For this review, take the finished solid that the model builds, in its own axes (mm). Face numbers are marked on the shaded views. Give positions to 0.01 mm unless a question says otherwise; leave off trailing zeros. Order: outer loops, then holes, each group sorted by start corner. A loop starts at its lowest first (then second) coordinate and runs counter-clockwise, first axis right, second up. Notation, with made-up numbers: M -34.5,21 L 15.5,21 A30 ccw 15.5,60 Z; hole C -4.75,11 d5. An arc over 180 degrees is marked long. Use CSV: the item, a comma, the result in double quotes. Start each with the question number.
(1) Clearance check with flat-ended pins moving along their axes: P1, Ø1.6, axis at x = -85.5, z = 3, coming from the -Y side; P2, Ø2.5, axis at x = 146, z = 2.5, coming from the +Y side; P3, Ø6, axis at x = 94, y = 28.5, coming from the -Z side; P4, Ø1.8, axis at x = -133.5, z = 1.5, coming from the +Y side. State where each tip first meets the part, or that it passes through.
(2) Wall thickness on L1, parallel to X at y = 31.5, z = 1.3; L2, parallel to X at y = 53, z = 4.7; L3, parallel to X at y = 70, z = 1.5: over which ranges is each line inside the solid? List them lowest first. Write a range as from..to.
(3) Consider section C-C (z = 3.8). Give the number of separate pieces and of enclosed holes in the cut face, and give its area (3 significant figures).
(4) Draft analysis for pull direction Z (two halves, no side actions). For the marked faces 1 and 2, state which applies: pulls with the +Z half, pulls with the -Z half, needs draft (parallel to the pull), parting line crosses it, or undercut.
(5) Consider section A-A (y = 11.5). Write out the cut boundary in (x, z), and give its area (3 significant figures).
(6) Consider section B-B (x = -23). Write out the cut boundary in (y, z), and give its area (3 significant figures).
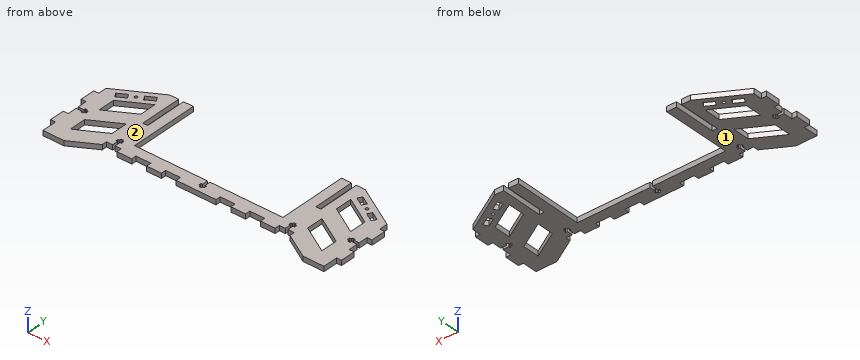
```python
from build123d import *

# Parameters (mm, degrees)
ESTRUSIONE_ESTRUSIONE1_DEPTH = 5
SCHIZZO2_R                   = 1.5
TAGLIO_ESTRUSIONE2_DEPTH     = 6
SCHIZZO5_W                   = 15
SCHIZZO5_H                   = 5
SCHIZZO5_W_2                 = 5
SCHIZZO5_H_2                 = 42.5
SCHIZZO5_W_3                 = 150.358983848
SCHIZZO5_H_3                 = 70
TAGLIO_ESTRUSIONE3_DEPTH     = 6
TAGLIO_ESTRUSIONE4_DEPTH     = 6
SCHIZZO7_R                   = 0.25
TAGLIO_ESTRUSIONE5_DEPTH     = 10


with BuildPart() as part:
    # Schizzo1 → Estrusione-Estrusione1 (new body)
    with BuildSketch(Plane.XY):
        Polygon((-142.5, 75), (-142.5, 66.339745962), (-147.5, 66.339745962), (-147.5, 51.339745962), (-142.5, 51.339745962), (-142.5, 30), (-147.5, 30), (-147.5, 15), (-142.5, 15), (-142.5, 0), (142.5, 0), (142.5, 15), (147.5, 15), (147.5, 30), (142.5, 30), (142.5, 51.339745962), (147.5, 51.339745962), (147.5, 66.339745962), (142.5, 66.339745962), (142.5, 75), (99.198729811, 100), (-99.198729811, 100), align=None)
    extrude(amount=ESTRUSIONE_ESTRUSIONE1_DEPTH)

    # Schizzo2 → Taglio-Estrusione2 (cut, through all)
    with BuildSketch(Plane.XY):
        with Locations((-117.099364905, 81.004809472)):
            Circle(SCHIZZO2_R)
        with Locations((117.099364905, 81.004809472)):
            Circle(SCHIZZO2_R)
        Polygon((-99.198729811, 82.679491924), (-127.5, 66.339745962), (-127.5, 49.330127019), (-99.198729811, 65.669872981), align=None)
        Polygon((99.198729811, 31.339745962), (99.198729811, 48.349364905), (127.5, 32.009618943), (127.5, 15), align=None)
        Polygon((-95.179491924, 15), (-121.160254038, 0), (121.160254038, 0), (95.179491924, 15), align=None)
        Polygon((-99.198729811, 31.339745962), (-127.5, 15), (-127.5, 32.009618943), (-99.198729811, 48.349364905), align=None)
        Polygon((99.198729811, 65.669872981), (99.198729811, 82.679491924), (127.5, 66.339745962), (127.5, 49.330127019), align=None)
        Polygon((-132.5, 75), (-123.839745962, 80), (-121.339745962, 75.669872981), (-130, 70.669872981), align=None)
        Polygon((-104.198729811, 91.339745962), (-101.698729811, 87.009618943), (-110.358983849, 82.009618943), (-112.858983849, 86.339745962), align=None)
        Polygon((132.5, 75), (130, 70.669872981), (121.339745962, 75.669872981), (123.839745962, 80), align=None)
        Polygon((104.198729811, 91.339745962), (112.858983849, 86.339745962), (110.358983849, 82.009618943), (101.698729811, 87.009618943), align=None)
    extrude(amount=TAGLIO_ESTRUSIONE2_DEPTH, mode=Mode.SUBTRACT)

    # Schizzo5 → Taglio-Estrusione3 (cut, through all)
    with BuildSketch(Plane.XY):
        with Locations((-87.679491924, 17.5)):
            Rectangle(SCHIZZO5_W, SCHIZZO5_H)
        with Locations((-57.679491924, 17.5)):
            Rectangle(SCHIZZO5_W, SCHIZZO5_H)
        with Locations((-27.679491924, 17.5)):
            Rectangle(SCHIZZO5_W, SCHIZZO5_H)
        with Locations((27.679491924, 17.5)):
            Rectangle(SCHIZZO5_W, SCHIZZO5_H)
        with Locations((57.679491924, 17.5)):
            Rectangle(SCHIZZO5_W, SCHIZZO5_H)
        with Locations((87.679491924, 17.5)):
            Rectangle(SCHIZZO5_W, SCHIZZO5_H)
        with Locations((87.679491924, 78.75)):
            Rectangle(SCHIZZO5_W_2, SCHIZZO5_H_2)
        with Locations((-87.679491924, 78.75)):
            Rectangle(SCHIZZO5_W_2, SCHIZZO5_H_2)
        with Locations((0, 65)):
            Rectangle(SCHIZZO5_W_3, SCHIZZO5_H_3)
    extrude(amount=TAGLIO_ESTRUSIONE3_DEPTH, mode=Mode.SUBTRACT)

    # Schizzo6 → Taglio-Estrusione4 (cut, through all)
    with BuildSketch(Plane.XY):
        Polygon((-142.5, 41.919872981), (-136.5, 41.919872981), (-136.5, 43.419872981), (-134.1, 43.419872981), (-134.1, 41.919872981), (-132.5, 41.919872981), (-132.5, 39.419872981), (-134.1, 39.419872981), (-134.1, 37.919872981), (-136.5, 37.919872981), (-136.5, 39.419872981), (-142.5, 39.419872981), align=None)
        Polygon((134.1, 43.419872981), (134.1, 41.919872981), (132.5, 41.919872981), (132.5, 39.419872981), (134.1, 39.419872981), (134.1, 37.919872981), (136.5, 37.919872981), (136.5, 39.419872981), (142.5, 39.419872981), (142.5, 41.919872981), (136.5, 41.919872981), (136.5, 43.419872981), align=None)
        Polygon((-88.929491924, 20), (-88.929491924, 26), (-90.429491924, 26), (-90.429491924, 28.4), (-88.929491924, 28.4), (-88.929491924, 30), (-86.429491924, 30), (-86.429491924, 28.4), (-84.929491924, 28.4), (-84.929491924, 26), (-86.429491924, 26), (-86.429491924, 20), align=None)
        Polygon((86.429491924, 20), (88.929491924, 20), (88.929491924, 26), (90.429491924, 26), (90.429491924, 28.4), (88.929491924, 28.4), (88.929491924, 30), (86.429491924, 30), (86.429491924, 28.4), (84.929491924, 28.4), (84.929491924, 26), (86.429491924, 26), align=None)
        Polygon((-1.25, 20), (-1.25, 21.6), (-2.75, 21.6), (-2.75, 24), (-1.25, 24), (-1.25, 30), (1.25, 30), (1.25, 24), (2.75, 24), (2.75, 21.6), (1.25, 21.6), (1.25, 20), align=None)
    extrude(amount=TAGLIO_ESTRUSIONE4_DEPTH, mode=Mode.SUBTRACT)

    # Schizzo7 → Taglio-Estrusione5 (cut)
    with BuildSketch(Plane.XY.offset(5)):
        with Locations((-136.5, 43.419872981)):
            Circle(SCHIZZO7_R)
        with Locations((-136.5, 37.919872981)):
            Circle(SCHIZZO7_R)
        with Locations((-90.429491924, 26)):
            Circle(SCHIZZO7_R)
        with Locations((-84.929491924, 26)):
            Circle(SCHIZZO7_R)
        with Locations((-2.75, 24)):
            Circle(SCHIZZO7_R)
        with Locations((2.75, 24)):
            Circle(SCHIZZO7_R)
        with Locations((84.929491924, 26)):
            Circle(SCHIZZO7_R)
        with Locations((90.429491924, 26)):
            Circle(SCHIZZO7_R)
        with Locations((136.5, 43.419872981)):
            Circle(SCHIZZO7_R)
        with Locations((136.5, 37.919872981)):
            Circle(SCHIZZO7_R)
    extrude(amount=-TAGLIO_ESTRUSIONE5_DEPTH, mode=Mode.SUBTRACT)


solid = part.part
```
Check result:
1,P1,"stops at y = 20"
1,P2,"stops at y = 66.34"
1,P3,"stops at z = 0"
1,P4,"stops at y = 80.72"
2,L1,"x = -142.5..-127.5, -99.2..-75.18, 75.18..99.2, 127.5..142.5"
2,L2,"x = -147.5..-127.5, -121.14..-75.18, 75.18..121.14, 127.5..147.5"
2,L3,"x = -142.5..-121.16, -99.2..-90.18, -85.18..-75.18, 75.18..85.18, 90.18..99.2, 121.16..142.5"
3,separate pieces,"1"
3,enclosed holes,"10"
3,area,"10,800 mm^2"
4,face 1,"pulls with the -Z half"
4,face 2,"pulls with the +Z half"
5,outline,"M -142.5,0 L -101.24,0 L -101.24,5 L -142.5,5 Z; M 101.24,0 L 142.5,0 L 142.5,5 L 101.24,5 Z"
5,area,"413 mm^2"
6,outline,"M 20,0 L 30,0 L 30,5 L 20,5 Z"
6,area,"50.0 mm^2"
